Can you work these out from the model? Positions are in its coordinate system, mm. A direction names the side the tool comes from. Round coordinates to 2 decimals unless told otherwise and drop trailing zeros. Loops run counter-clockwise (first coordinate to the right, second up) from the corner with the lowest first, then second, coordinate; pieces in that order, holes last.
(1) I want a section at C-C on x = 47. Write out the boundary of the cut face in (y, z).
(2) Will this pin go through, and if not, where does the flat tip stop? pin 1 Ø12 at (x, z) = (76, 16.5) entering from +Y.
(3) I want a section at A-A on y = 8.5. Write out the boundary of the cut face in (x, z), plus the area to 3 significant figures.
(4) If I drill on line 1 along Z through (x, y) = (65.5, 5.5); line 2 along X through (y, z) = (4, 24); line 3 along Y through (x, z) = (68.5, 5), over which ranges is the centre line in solid material (lowest first)?
(5) I want a section at B-B on z = 5.5. Write out the boundary of the cut face in (x, y), plus the area to 3 significant figures.
(6) Thinking about a two-plate mould opening in Z: for faces 4 (the face through (48, 7, 25)), 5 (the face through (47, 10, -3)), 6 (the face through (44, 20, 26)), which applies, released by +Z, released by -Z, zero draft, split by the parting line, or undercut?
(7) Which directions (+Z, -Z, +X, -X, +Y, -Y) give clear straight access to the entire face, cutting with the end or side of a thin tool? Please do faces 1 (the face through (46.84, 12.71, 25.98)), 2 (the face through (47, 17, 0)), 3 (the face through (-3, 10, 13)).
Autodesk Fusion 360 part; units mm, degrees
sketch "Sketch1" plane through (0, 0, 0) normal (0, 1, 0) x (1, 0, 0)
  line L0 (0, 0) -> (95, 0)
  line L1 (95, 0) -> (95, -25)
  line L2 (95, -25) -> (0, -25)
  line L3 (0, -25) -> (0, 0)
  line L4 (98, 3) -> (98, -28)
  line L5 (98, -28) -> (-3, -28)
  line L6 (-3, -28) -> (-3, 3)
  line L7 (-3, 3) -> (98, 3)
  dimension "d1" = 95
  dimension "d2" = 25
  dimension "d3" = -3
extrude "Extrude1" add sketch "Sketch1" along normal blind 20 makes body 1
extrude "Extrude2" add sketch "Sketch1" along normal blind 3 contours L0 L1 L2 L3 bodies 1
ref_plane "WorkPlane1" through (47.5, 10, 12.5) normal (0, 0, 1) x (1, 0, 0)
ref_plane "WorkPlane2" through (47.5, 10, 12.5) normal (1, 0, 0) x (0, 0, -1)
sketch "Sketch3" plane through (47.5, 0, 0) normal (1, 0, 0) x (0, 1, 0)
  line L0 (20, 28) -> (0, 28)
  line L1 (0, 28) -> (0, -3)
  line L2 (0, -3) -> (20, -3)
  line L3 (20, -3) -> (20, 0)
  line L4 (20, 0) -> (3, 0)
  line L5 (3, 0) -> (3, 25)
  line L6 (3, 25) -> (20, 25)
  line L7 (20, 25) -> (20, 28)
  circle A0 centre (12.8865, 25) radius 0.75
  circle A1 centre (12.8865, 25) radius 0.9942
  arc A2 (12.1481, 24.8686) -> (20, 21.2966) centre (16.9616, 25.0336) ccw
  arc A3 (13.6365, 25) -> (20, 25) centre (16.8183, 27.2777) ccw
  line L8 (23.2, 12.5) -> (-3.2, 12.5)
  line L9 (20, 28) -> (20, -3)
  line L10 (20, 28) -> (16, 28)
  line L11 (16, 28) -> (16, -3)
  line L12 (20, -3) -> (16, -3)
  arc A4 (20, 0) -> (13.6365, 0) centre (16.8183, -2.2777) ccw
  arc A5 (20, 3.7034) -> (12.1481, 0.1314) centre (16.9616, -0.0336) ccw
  circle A6 centre (12.8865, 0) radius 0.75
  circle A7 centre (12.8865, 0) radius 0.9942
  dimension "d8" = 1.5
extrude "Extrude9" cut sketch "Sketch3" along normal mid plane 95 contours L6 A1 A3 | L6 A0 A1 | A0 A1 A2 A3 | L6 A0 | L6 A0 | L6 A0 A1 A2 | L4 A5 A6 A7 | L4 A6 A7 | A4 A5 A6 A7 | L4 A4 A7 | L4 A6 | L4 A6 bodies 1
extrude "Extrude10" add sketch "Sketch3" along normal blind 4 from surface at 20 separate body contours A2 A3 L9 L11 | A1 A2 A3 L11 | A0 A1 A2 A3 | L6 A0 | L6 A0 | L9 L11 A4 A5 | L11 A4 A5 A7 | A4 A5 A6 A7 | L4 A6 | L4 A6 makes body 2 at (70.1667, 12.334, 23.6987) makes body 3 at (70.1667, 18.5562, 4.5111)
extrude "Extrude11" add sketch "Sketch3" along normal blind 4 from surface at -20 separate body contours A2 A3 L9 L11 | A1 A2 A3 L11 | A0 A1 A2 A3 | L6 A0 | L6 A0 | L9 L11 A4 A5 | L11 A4 A5 A7 | A4 A5 A6 A7 | L4 A6 | L4 A6 makes body 4 at (30.1667, 18.5562, 4.5111) makes body 5 at (30.1667, 12.334, 23.6987)
extrude "Extrude12" add sketch "Sketch3" along normal mid plane 101 separate body contours L0 L6 L7 L9 L10 L11 | L6 A3 L11 | A2 A3 L9 L11 | A2 L8 L9 L11 | L8 L9 L11 A5 | L9 L11 A4 A5 | L2 L3 L4 L9 L11 L12 | L4 L11 A4 makes body 6
sketch "Sketch8" plane through (0, 16, 0) normal (0, -1, 0) x (1, 0, 0)
  line L0 (-3, -3) -> (98, -3)
  line L1 (98, -3) -> (98, 28)
  line L2 (98, 28) -> (-3, 28)
  line L3 (-3, 28) -> (-3, -3)
  line L4 (0, 10) -> (2.4867, 10)
  line L5 (2.4867, 10) -> (2.4867, 15)
  line L6 (2.4867, 15) -> (0, 15)
  line L7 (0, 15) -> (0, 10)
  line L8 (95, 10) -> (93, 10)
  line L9 (93, 10) -> (93, 15)
  line L10 (93, 15) -> (95, 15)
  line L11 (95, 10) -> (95, 15)
extrude "Extrude13" add sketch "Sketch8" along normal blind 2 contours L4 L5 L6 L7 | L8 L9 L10 L11 bodies 6
fillet "Fillet5" radius 0.5 4 edges at (47.5, 20, 28) (98, 20, 12.5) (47.5, 20, -3) (-3, 20, 12.5) on bodies 6
fillet "Fillet6" radius 1 2 edges at (47.5, 13.8807, 25) (47.5, 13.8807, 0) on bodies 1
fillet "Fillet7" radius 0.5 8 edges at (-3, 10, 28) (-3, 0, 12.5) (-3, 10, -3) (47.5, 0, -3) (47.5, 0, 28) (98, 0, 12.5) (98, 10, -3) (98, 10, 28) on bodies 1
fillet "Fillet8" radius 0.25 2 edges at (47.5, 11.8923, 0) (47.5, 11.8923, 25) on bodies 1
fillet "Fillet9" radius 0.5 4 edges at (47.5, 20, 0) (0, 20, 12.5) (47.5, 20, 25) (95, 20, 12.5) on bodies 1
hidden bodies 2 3 5 4 6
Filled sheet:
1. outline: (0, -2.5) arc R0.5 ccw to (0.5, -3) - (20, -3) - (20, -0.5) arc R0.5 ccw to (19.5, 0) - (14.61, 0) arc R1 ccw to (13.75, -0.5) arc R0.99 cw to (11.91, -0.2) arc R0.25 ccw to (11.67, 0) - (3, 0) - (3, 25) - (11.67, 25) arc R0.25 ccw to (11.91, 25.2) arc R0.99 cw to (13.75, 25.5) arc R1 ccw to (14.61, 25) - (19.5, 25) arc R0.5 ccw to (20, 25.5) - (20, 28) - (0.5, 28) arc R0.5 ccw to (0, 27.5) - close
2. pin 1: stops at y = 3
3. outline: (-3, -2.5) arc R0.5 ccw to (-2.5, -3) - (97.5, -3) arc R0.5 ccw to (98, -2.5) - (98, 27.5) arc R0.5 ccw to (97.5, 28) - (-2.5, 28) arc R0.5 ccw to (-3, 27.5) - close; hole (0, 0) - (95, 0) - (95, 25) - (0, 25) - close
3. area: 756 mm2
4. line 1: z = -3 to 0, 25 to 28
4. line 2: x = -3 to 0, 95 to 98
4. line 3: y = 0 to 3
5. outline: (-3, 0.5) arc R0.5 ccw to (-2.5, 0) - (97.5, 0) arc R0.5 ccw to (98, 0.5) - (98, 20) - (95.5, 20) arc R0.5 ccw to (95, 19.5) - (95, 3) - (0, 3) - (0, 19.5) arc R0.5 ccw to (-0.5, 20) - (-3, 20) - close
5. area: 405 mm2
6. face 4: undercut
6. face 5: released by -Z
6. face 6: zero draft
7. face 1: none
7. face 2: +Y
7. face 3: +Z, -Z, -X, +Y, -Y
